from build123d import *

# Parameters (mm, degrees)
PIPE_CONNECTOR_FILLET_R = 5


with BuildPart() as part:
    # Sketch1 → Revolve1 (revolve)
    with BuildSketch(Plane.XY):
        with BuildLine():
            Line((-225, 175), (225, 175))
            ThreePointArc((225, 175), (242.67766953, 167.67766953), (250, 150))
            Line((250, 150), (250, 35))
            Line((250, 35), (310, 35))
            Line((310, 35), (310, 25))
            Line((310, 25), (225, 25))
            Line((225, 25), (225, 137.5))
            ThreePointArc((225, 137.5), (221.338834765, 146.338834765), (212.5, 150))
            Line((212.5, 150), (-212.5, 150))
            ThreePointArc((-212.5, 150), (-221.338834765, 146.338834765), (-225, 137.5))
            Line((-225, 137.5), (-225, 0))
            Line((-225, 0), (-250, 0))
            Line((-250, 0), (-250, 150))
            ThreePointArc((-250, 150), (-242.67766953, 167.67766953), (-225, 175))
        make_face()
    revolve(axis=Axis((-162.28666216, 0, 0), (1, 0, 0)))

    # Pipe Connector Fillet
    pipe_connector_fillet_edges = [part.edges().sort_by_distance(p)[0] for p in [
        (250, -35, 0),
    ]]
    fillet(pipe_connector_fillet_edges, radius=PIPE_CONNECTOR_FILLET_R)


solid = part.part
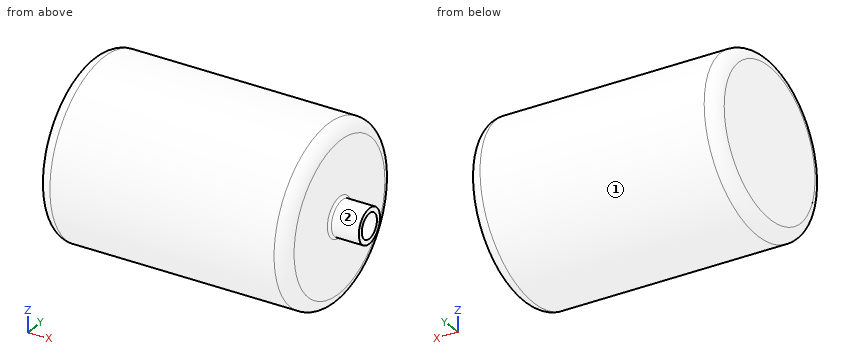
The listing builds one solid part. Answer for the finished solid, in the listing's coordinates (mm). Face numbers are marked on the shaded views. A direction names the side the tool comes from. Give positions to 0.01 mm unless a question says otherwise; leave off trailing zeros. Write each loop counter-clockwise with the first axis right and the second up, starting at its lowest first coordinate (ties: lowest second). Pieces come first, ordered by that corner, then holes. Notation, with made-up numbers: (18, 14) - (50, 14) arc R13 cw to (50, 29) - close; hole circle Ø4 at (87.5, 14). An arc over 180 degrees is marked (long way). Use a Markdown table: item, result.
1. Each of these flat-tipped pins is pushed along its axis until it touches: P1, Ø3, axis at x = 167, z = 93, coming from the -Y side; P2, Ø5, axis at y = -100, z = 70.5, coming from the +X side; P3, Ø4, axis at x = 39, z = 32, coming from the +Y side. Where does it stop, or does it pass through?
Values follow:
| item | result |
|---|---|
| P1 | stops at y = -149.17 |
| P2 | stops at x = 250 |
| P3 | stops at y = 172.41 |
2. Section C-C on x = -110 is taken. Write down the section's boundary in (y, z).
Values follow:
| item | result |
|---|---|
| outline | circle Ø350 at (0, 0); hole circle Ø300 at (0, 0) |
3. A tool of negligible diameter and unlimited length cuts with its end or side. For the marked faces 1 and 2, from which of +Z, -Z, +X, -X, +Y, -Y can it reach the whole face along a straight path? Write none if from no direction.
Values follow:
| item | result |
|---|---|
| face 1 | +X, -X |
| face 2 | +X |
4. Section A-A on z = 0 is taken. Write down the section's boundary in (x, y).
Values follow:
| item | result |
|---|---|
| outline | (-250, -150) arc R25 ccw to (-225, -175) - (225, -175) arc R25 ccw to (250, -150) - (250, -40) arc R5 cw to (255, -35) - (310, -35) - (310, -25) - (225, -25) - (225, -137.5) arc R12.5 cw to (212.5, -150) - (-212.5, -150) arc R12.5 cw to (-225, -137.5) - (-225, 137.5) arc R12.5 cw to (-212.5, 150) - (212.5, 150) arc R12.5 cw to (225, 137.5) - (225, 25) - (310, 25) - (310, 35) - (255, 35) arc R5 cw to (250, 40) - (250, 150) arc R25 ccw to (225, 175) - (-225, 175) arc R25 ccw to (-250, 150) - close |
5. Find the intervals of material crossed by probe 1 along Z at (x, y) = (276, 0); probe 2 along X at (y, z) = (80.5, 28.5); probe 3 along Z at (x, y) = (-29, 0), in increasing order. Write a range as from..to.
Values follow:
| item | result |
|---|---|
| probe 1 | z = -35..-25, 25..35 |
| probe 2 | x = -250..-225, 225..250 |
| probe 3 | z = -175..-150, 150..175 |
6. Section D-D on x = 272.5 is taken. Write down the section's boundary in (y, z), plus the area to 3 significant figures.
Values follow:
| item | result |
|---|---|
| outline | circle Ø70 at (0, 0); hole circle Ø50 at (0, 0) |
| area | 1,880 mm² |
